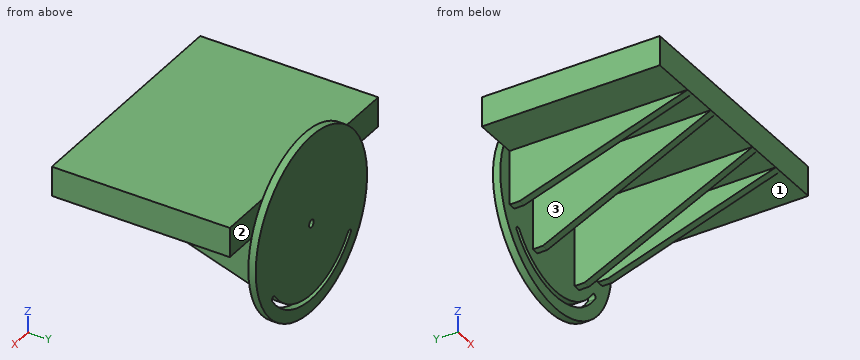
from build123d import *

# Parameters (mm, degrees)
F0_R      = 228.6
F1_DEPTH  = 19.05
F2_W      = 19.05
F2_H      = 139.7
F2_H_2    = 203.2
F3_DEPTH  = 457.2
F5_DEPTH  = 25.4
F7_DEPTH  = 25.4
F9_DEPTH  = 25.4
F11_DEPTH = 25.4


with BuildPart() as f1:
    # F0 (on Front) → F1 (new body)
    with BuildSketch(Plane.XZ):
        Circle(F0_R)
        with BuildLine():
            ThreePointArc((161.25008, -112.908521), (0, -196.85), (-161.25008, -112.908521))
            ThreePointArc((-161.25008, -112.908521), (-159.690675, -104.064696), (-150.846849, -105.624101))
            ThreePointArc((-150.846849, -105.624101), (0, -184.15), (150.846849, -105.624101))
            ThreePointArc((150.846849, -105.624101), (159.690675, -104.064696), (161.25008, -112.908521))
        make_face(mode=Mode.SUBTRACT)
        with BuildLine():
            ThreePointArc((-7.802423, -5.463316), (-2.864223, 9.084154), (9.525, 0))
            ThreePointArc((9.525, 0), (9.084154, -2.864223), (7.802423, -5.463316))
            ThreePointArc((7.802423, -5.463316), (4.398156, -8.448778), (0, -9.525))
            ThreePointArc((0, -9.525), (-4.398156, -8.448778), (-7.802423, -5.463316))
        make_face(mode=Mode.SUBTRACT)
    extrude(amount=F1_DEPTH)

    # F2 (on face) → F3 (join)
    with BuildSketch(Plane.XZ.offset(19.05)):
        with BuildLine():
            Line((304.8, 152.4), (170.38838, 152.4))
            ThreePointArc((170.38838, 152.4), (196.682779, 116.506843), (215.526147, 76.2))
            Line((215.526147, 76.2), (304.8, 76.2))
            Line((304.8, 76.2), (304.8, 152.4))
        make_face()
        with BuildLine():
            Line((170.38838, 152.4), (-170.38838, 152.4))
            ThreePointArc((-170.38838, 152.4), (-196.682779, 116.506843), (-215.526147, 76.2))
            Line((-215.526147, 76.2), (-190.5, 76.2))
            Line((-190.5, 76.2), (-171.45, 76.2))
            Line((-171.45, 76.2), (-95.25, 76.2))
            Line((-95.25, 76.2), (-76.2, 76.2))
            Line((-76.2, 76.2), (76.2, 76.2))
            Line((76.2, 76.2), (95.25, 76.2))
            Line((95.25, 76.2), (171.45, 76.2))
            Line((171.45, 76.2), (190.5, 76.2))
            Line((190.5, 76.2), (215.526147, 76.2))
            ThreePointArc((215.526147, 76.2), (196.682779, 116.506843), (170.38838, 152.4))
        make_face()
        with BuildLine():
            Line((-170.38838, 152.4), (-304.8, 152.4))
            Line((-304.8, 152.4), (-304.8, 76.2))
            Line((-304.8, 76.2), (-215.526147, 76.2))
            ThreePointArc((-215.526147, 76.2), (-196.682779, 116.506843), (-170.38838, 152.4))
        make_face()
        with Locations((-180.975, 6.35)):
            Rectangle(F2_W, F2_H)
        with Locations((-85.725, -25.4)):
            Rectangle(F2_W, F2_H_2)
        with Locations((85.725, -25.4)):
            Rectangle(F2_W, F2_H_2)
        with Locations((180.975, 6.35)):
            Rectangle(F2_W, F2_H)
    extrude(amount=F3_DEPTH)

    # F4 (on face) → F5 (cut)
    with BuildSketch(Plane.YZ.offset(190.5)):
        Polygon((-44.45, -63.5), (-476.25, 76.2), (-476.25, -63.5), align=None)
    extrude(amount=-F5_DEPTH, mode=Mode.SUBTRACT)

    # F6 (on face) → F7 (cut)
    with BuildSketch(Plane.YZ.offset(95.25)):
        Polygon((-44.45, -127), (-476.25, 76.2), (-476.25, -127), align=None)
    extrude(amount=-F7_DEPTH, mode=Mode.SUBTRACT)

    # F8 (on face) → F9 (cut)
    with BuildSketch(Plane.YZ.offset(-76.2)):
        Polygon((-44.45, -127), (-476.25, 76.2), (-476.25, -127), align=None)
    extrude(amount=-F9_DEPTH, mode=Mode.SUBTRACT)

    # F10 (on face) → F11 (cut)
    with BuildSketch(Plane(origin=(-190.5, 0, 0), x_dir=(0, -1, 0), z_dir=(-1, 0, 0))):
        Polygon((476.25, -63.5), (476.25, 76.2), (44.45, -63.5), align=None)
    extrude(amount=-F11_DEPTH, mode=Mode.SUBTRACT)


solid = f1.part
Could you check a few things on this model? Use its own coordinates, in mm. Face numbers are marked on the shaded views. A direction names the side the tool comes from. Round coordinates to 2 decimals unless told otherwise and drop trailing zeros. Order: outer loops, then holes, each group sorted by start corner. A loop starts at its lowest first (then second) coordinate and runs counter-clockwise, first axis right, second up.
(1) Please list where these lines run through material, in increasing order: line 1 along X through (y, z) = (-71.5, 12.5); line 2 along X through (y, z) = (-46.5, -95); line 3 along Y through (x, z) = (-140, -151).
Response values:
line 1: x = -190.5 to -171.45, -95.25 to -76.2, 76.2 to 95.25, 171.45 to 190.5
line 2: x = -95.25 to -76.2, 76.2 to 95.25
line 3: y = -19.05 to 0
(2) Imagine slicing it at A-A (x = -25). Write out the boundary of the cut face in (y, z), plus the area to 3 significant figures.
Response values:
outline: (-476.25, 76.2) - (-19.05, 76.2) - (-19.05, -182.45) - (0, -182.45) - (0, 227.23) - (-19.05, 227.23) - (-19.05, 152.4) - (-476.25, 152.4) - close; (-19.05, -227.23) - (0, -227.23) - (0, -195.26) - (-19.05, -195.26) - close
area: 43,300 mm2
(3) Imagine slicing it at C-C (z = 44.5). Write out the boundary of the cut face in (x, y), plus the area to 3 significant figures.
Response values:
outline: (-224.23, -19.05) - (-190.5, -19.05) - (-190.5, -378.27) - (-171.45, -378.27) - (-171.45, -19.05) - (-95.25, -19.05) - (-95.25, -408.89) - (-76.2, -408.89) - (-76.2, -19.05) - (76.2, -19.05) - (76.2, -408.89) - (95.25, -408.89) - (95.25, -19.05) - (171.45, -19.05) - (171.45, -378.27) - (190.5, -378.27) - (190.5, -19.05) - (224.23, -19.05) - (224.23, 0) - (-224.23, 0) - close
area: 37,100 mm2
(4) Imagine slicing it at B-B (y = -352). Write out the boundary of the cut face in (x, z), plus the area to 3 significant figures.
Response values:
outline: (-304.8, 76.2) - (-190.5, 76.2) - (-190.5, 36) - (-171.45, 36) - (-171.45, 76.2) - (-95.25, 76.2) - (-95.25, 17.73) - (-76.2, 17.73) - (-76.2, 76.2) - (76.2, 76.2) - (76.2, 17.73) - (95.25, 17.73) - (95.25, 76.2) - (171.45, 76.2) - (171.45, 36) - (190.5, 36) - (190.5, 76.2) - (304.8, 76.2) - (304.8, 152.4) - (-304.8, 152.4) - close
area: 50,200 mm2
(5) I'm going to push flat-ended pins straight in: pin 1 (9.5 mm diameter, centred on x = 89, y = -31, fed in from -Z); pin 2 (10 mm diameter, centred on y = -185.5, z = 28.5, fed in from +X); pin 3 (6 mm diameter, centred on x = -0.5, y = -342.5, fed in from +Z). Where does each tip first touch, or does it pass through?
Response values:
pin 1: stops at z = -127
pin 2: stops at x = 190.5
pin 3: stops at z = 152.4
(6) Which directions (+Z, -Z, +X, -X, +Y, -Y) give clear straight access to the entire face, cutting with the end or side of a thin tool? Please do the marked faces 1, 2 and 3.
Response values:
face 1: -Z, +X, -Y
face 2: +Z, +X, +Y
face 3: -Z, -Y
